Verification items for this drawing (mm, ordinates from the low corner). A direction names the side the tool comes from. Round coordinates to 2 decimals unless told otherwise and drop trailing zeros. Order: outer loops, then holes, each group sorted by start corner. A loop starts at its lowest first (then second) coordinate and runs counter-clockwise, first axis right, second up. Notation, with made-up numbers: (11.5, 41) -> (16.5, 41) arc R35 ccw to (16.5, 77) -> close; hole circle Ø3 at (-6, -17). An arc over 180 degrees is marked (long way). Answer in a Markdown table with one row per item. Add a question column.
1. Material ranges on L1, parallel to Y at x = 2.5, z = 7.75; L2, parallel to X at y = 16.5, z = 9; L3, parallel to Z at x = 7.75, y = 20.25 (1 decimal), recorded low to high. Write a range as from..to.
2. Draft check along Y on the marked faces 1, 2, 3 and 4. Enter one of: +Y half, -Y half, draft (parallel to the pull), parting line (faces both ways), or undercut.
3. Sectioned sample at A-A, the plane x = 1. Count the separate pieces of the cut face and the enclosed holes in it, then the cut area to 3 significant figures.
4. Sectioned sample at C-C, the plane z = 1. Record the boundary of the cut face in (x, y).
5. Sectioned sample at D-D, the plane y = 16. Record the boundary of the cut face in (x, z), then the cut area to 3 significant figures.
6. Access from +Z, -Z, +X, -X, +Y, -Y to the whole of each face (thin tool, end or side, straight path). Record for the marked faces 5, 6, 7, 8 and 9.
7. Sectioned sample at B-B, the plane y = 19.5. Record the boundary of the cut face in (x, z).
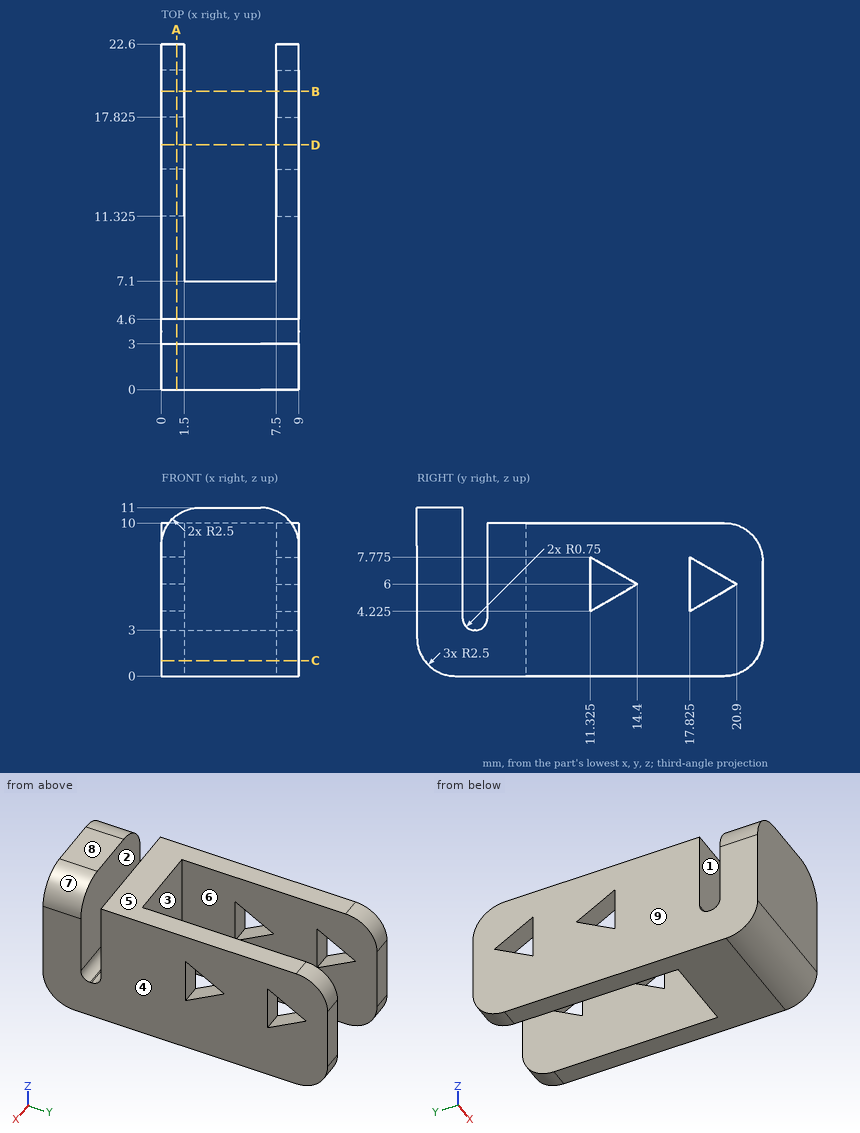
Answer key:
| question | item | result |
|---|---|---|
| 1 | L1 | y = 0..3, 4.6..7.1 |
| 1 | L2 | x = 0..1.5, 7.5..9 |
| 1 | L3 | z = 0..5.6, 6.4..10 |
| 2 | face 1 | undercut |
| 2 | face 2 | undercut |
| 2 | face 3 | +Y half |
| 2 | face 4 | draft |
| 3 | separate pieces | 1 |
| 3 | enclosed holes | 2 |
| 3 | area | 202 mm² |
| 4 | outline | (0, 0.5) -> (9, 0.5) -> (9, 22.1) -> (7.5, 22.1) -> (7.5, 7.1) -> (1.5, 7.1) -> (1.5, 22.1) -> (0, 22.1) -> close |
| 5 | outline | (0, 0) -> (1.5, 0) -> (1.5, 10) -> (0, 10) -> close; (7.5, 0) -> (9, 0) -> (9, 10) -> (7.5, 10) -> close |
| 5 | area | 30.0 mm² |
| 6 | face 5 | +Z, +X, -X, +Y |
| 6 | face 6 | +Z, -Z, +Y |
| 6 | face 7 | +Z, +X, -Y |
| 6 | face 8 | +Z, +X, -X, +Y, -Y |
| 6 | face 9 | +Z, -Z, -X, +Y, -Y |
| 7 | outline | (0, 0) -> (1.5, 0) -> (1.5, 5.19) -> (0, 5.19) -> close; (0, 6.81) -> (1.5, 6.81) -> (1.5, 10) -> (0, 10) -> close; (7.5, 0) -> (9, 0) -> (9, 5.19) -> (7.5, 5.19) -> close; (7.5, 6.81) -> (9, 6.81) -> (9, 10) -> (7.5, 10) -> close |
